Read the model definition and answer for the solid it produces. Units are mm, in the model's axes. Give positions to 0.01 mm unless a question says otherwise; leave off trailing zeros.
Autodesk Inventor part; units mm, degrees
ref_plane "YZ Plane" through (0, 0, 0) normal (1, 0, 0) x (0, 1, 0)
ref_plane "XZ Plane" through (0, 0, 0) normal (0, 1, 0) x (-1, 0, 0)
ref_plane "XY Plane" through (0, 0, 0) normal (0, 0, 1) x (1, 0, 0)
sketch "Sketch1" plane through (0, 0, 0) normal (0, 1, 0) x (-1, 0, 0)
  line L0 (69.85, 76.2) -> (-69.85, 76.2)
  line L1 (-69.85, 76.2) -> (-69.85, -76.2)
  line L2 (-69.85, -76.2) -> (69.85, -76.2)
  line L3 (69.85, -76.2) -> (69.85, 76.2)
  point P0 (0, 0)
  dimension "d0" = 152.4
  dimension "d1" = 139.7
  dimension "d2" = 69.85
  dimension "d3" = 76.2
extrude "Extrusion1" add sketch "Sketch1" along normal blind 12.7
sketch "Sketch4" plane through (0, 12.7, 0) normal (0, 1, 0) x (1, 0, 0)
  circle A0 centre (63.5, 69.85) radius 3.175
  circle A1 centre (63.5, -69.85) radius 3.175
  circle A2 centre (-60.96, -52.07) radius 3.175
  line L0 (69.85, 76.2) -> (-69.85, 76.2)
  line L1 (69.85, -76.2) -> (69.85, 76.2)
  line L2 (-69.85, -76.2) -> (69.85, -76.2)
  line L3 (-69.85, 76.2) -> (-69.85, -76.2)
  circle A3 centre (-60.96, 52.07) radius 3.175
  point P0 (0, 0)
  dimension "d20" = 6.35
  dimension "d21" = 6.35
  dimension "d22" = 6.35
  dimension "d23" = 6.35
  dimension "d24" = 6.35
  dimension "d25" = 6.35
  dimension "d26" = 6.35
  dimension "d27" = 24.13
  dimension "d28" = 8.89
  dimension "d32" = 6.35
  dimension "d33" = 24.13
  dimension "d34" = 8.89
extrude "Extrusion6" [suppressed]
fillet "Fillet1" [suppressed]
sketch "Sketch7" plane through (0, 12.7, 0) normal (0, 1, 0) x (1, 0, 0)
  arc A0 (-69.85, -37.0366) -> (-18.2851, -76.2) centre (46.0045, 61.976) ccw
  line L0 (69.85, 76.2) -> (-69.85, 76.2)
  line L1 (69.85, -76.2) -> (69.85, 76.2)
  line L2 (-69.85, 76.2) -> (-69.85, -76.2)
  line L3 (-69.85, -76.2) -> (69.85, -76.2)
  line L4 (-69.85, 76.2) -> (-69.85, -76.2)
  arc A1 (-18.2851, -76.2) -> (-69.85, -37.0366) centre (46.0045, 61.976) ccw
  point P0 (0, 0)
  point P1 (76.2, -60.325)
  point P2 (73.025, -60.325)
  point P3 (73.025, 63.5)
  point P4 (73.025, 60.325)
  point P5 (-73.025, 63.5)
  point P6 (76.2, 60.325)
  point P7 (73.025, -63.5)
  point P8 (-76.2, 60.325)
  point P9 (-80.9955, -22.2663)
  dimension "d46" = 304.8
  dimension "d47" = 14.224
  dimension "d48" = 23.8455
sketch "Sketch8" plane through (0, 12.7, 0) normal (0, 1, 0) x (1, 0, 0)
  circle A0 centre (-47.526, 0.6694) radius 1.4224
  circle A1 centre (-47.526, 0.6694) radius 1.4224
  circle A2 centre (-38.506, 0.6694) radius 1.4224
  line L0 (-33.996, -2.3847) -> (-52.036, -2.3847)
  line L1 (-33.996, 3.7235) -> (-33.996, -2.3847)
  line L2 (-33.996, 3.7235) -> (-52.036, 3.7235)
  line L3 (-52.036, -2.3847) -> (-52.036, 3.7235)
  circle A3 centre (-47.526, 33.9312) radius 1.4224
  circle A4 centre (-38.506, 33.9312) radius 1.4224
  line L4 (-33.996, 30.877) -> (-52.036, 30.877)
  line L5 (-33.996, 36.9853) -> (-33.996, 30.877)
  line L6 (-33.996, 36.9853) -> (-52.036, 36.9853)
  line L7 (-52.036, 30.877) -> (-52.036, 36.9853)
  circle A5 centre (2.54, -39.6875) radius 3.175 construction
  circle A6 centre (2.54, 12.7127) radius 3.175 construction
  circle A7 centre (2.54, 65.1129) radius 3.175 construction
  circle A8 centre (68.58, 65.1129) radius 3.175 construction
  circle A9 centre (68.58, 12.7127) radius 3.175 construction
  circle A10 centre (68.58, -39.6875) radius 3.175 construction
  circle A11 centre (-32.4275, -33.782) radius 1.4224
  circle A12 centre (-39.1585, -27.051) radius 1.4224
  circle A13 centre (-45.8895, -33.782) radius 1.4224
  circle A14 centre (-45.8895, 67.818) radius 1.4224
  circle A15 centre (-39.1585, 61.087) radius 1.4224
  circle A16 centre (-32.4275, 67.818) radius 1.4224
extrude "Extrusion9" cut sketch "Sketch8" against normal through all contours A0 | A2 | A3 | A4 | A11 | A12 | A13 | A14 | A15 | A16
extrude "Extrusion11" cut sketch "Sketch7" against normal through all contours A0 L3 L2
sketch "Sketch10" plane through (0, 12.7, 0) normal (0, 1, 0) x (1, 0, 0)
  circle A0 centre (62.611, 72.39) radius 1.4732
  arc A1 (-69.85, -37.0366) -> (-18.2851, -76.2) centre (46.0045, 61.976) ccw
  line L0 (-18.2851, -76.2) -> (69.85, -76.2)
  line L1 (69.85, -76.2) -> (69.85, 76.2)
  line L2 (69.85, 76.2) -> (-69.85, 76.2)
  line L3 (-69.85, 76.2) -> (-69.85, -37.0366)
  circle A2 centre (-47.526, 33.9312) radius 1.4224
  circle A3 centre (-47.526, 0.6694) radius 1.4224
  circle A4 centre (-38.506, 0.6694) radius 1.4224
  circle A5 centre (-38.506, 33.9312) radius 1.4224
  circle A6 centre (33.655, 72.39) radius 1.4732
  circle A7 centre (48.133, 72.39) radius 1.4732
  circle A8 centre (19.177, 72.39) radius 1.4732
  circle A9 centre (4.699, 72.39) radius 1.4732
  circle A10 centre (62.611, -68.58) radius 1.4732
  circle A11 centre (48.133, -68.58) radius 1.4732
  circle A12 centre (33.655, -68.58) radius 1.4732
  circle A13 centre (19.177, -68.58) radius 1.4732
  circle A14 centre (4.699, -68.58) radius 1.4732
  point P0 (0, 0)
extrude "Extrusion13" cut sketch "Sketch10" against normal through all contours A0 | A6 | A7 | A8 | A9 | A10 | A11 | A12 | A13 | A14
sketch "Sketch11" plane through (0, 12.7, 0) normal (0, 1, 0) x (1, 0, 0)
  circle A0 centre (19.177, 72.39) radius 1.4732
  circle A1 centre (48.133, 72.39) radius 1.4732
  circle A2 centre (62.611, -68.58) radius 1.4732
  circle A3 centre (33.655, -68.58) radius 1.4732
  circle A4 centre (4.699, -68.58) radius 1.4732
  circle A5 centre (1.27, -42.545) radius 1.4732
  circle A6 centre (1.27, -12.9117) radius 1.4732
  circle A7 centre (1.27, 16.7217) radius 1.4732
  circle A8 centre (1.27, 46.355) radius 1.4732
  circle A9 centre (66.04, 61.1717) radius 1.4732
  circle A10 centre (66.04, 31.5383) radius 1.4732
  circle A11 centre (66.04, 1.905) radius 1.4732
  circle A12 centre (66.04, -27.7283) radius 1.4732
  circle A13 centre (66.04, -57.3617) radius 1.4732
  circle A14 centre (66.04, -42.545) radius 1.4732
  circle A15 centre (66.04, -12.9117) radius 1.4732
  circle A16 centre (66.04, 16.7217) radius 1.4732
  circle A17 centre (66.04, 46.355) radius 1.4732
  circle A18 centre (1.27, 61.1717) radius 1.4732
  circle A19 centre (1.27, 31.5383) radius 1.4732
  circle A20 centre (1.27, 1.905) radius 1.4732
  circle A21 centre (1.27, -27.7283) radius 1.4732
  circle A22 centre (1.27, -57.3617) radius 1.4732
  circle A23 centre (19.177, -68.58) radius 1.4732
  circle A24 centre (48.133, -68.58) radius 1.4732
  circle A25 centre (62.611, 72.39) radius 1.4732
  circle A26 centre (33.655, 72.39) radius 1.4732
  circle A27 centre (4.699, 72.39) radius 1.4732
  line L0 (0.635, -72.39) -> (66.675, -72.39)
  line L1 (69.85, -69.215) -> (69.85, 73.025)
  line L2 (66.675, 76.2) -> (0.635, 76.2)
  line L3 (-2.54, 73.025) -> (-2.54, -69.215)
  arc A28 (59.055, 62.23) -> (55.88, 65.405) centre (55.88, 62.23) ccw
  line L4 (59.055, -58.42) -> (59.055, 62.23)
  arc A29 (55.88, -61.595) -> (59.055, -58.42) centre (55.88, -58.42) ccw
  line L5 (11.43, -61.595) -> (55.88, -61.595)
  arc A30 (8.255, -58.42) -> (11.43, -61.595) centre (11.43, -58.42) ccw
  line L6 (8.255, 62.23) -> (8.255, -58.42)
  arc A31 (11.43, 65.405) -> (8.255, 62.23) centre (11.43, 62.23) ccw
  line L7 (55.88, 65.405) -> (11.43, 65.405)
  arc A32 (69.85, 73.025) -> (66.675, 76.2) centre (66.675, 73.025) ccw
  arc A33 (0.635, 76.2) -> (-2.54, 73.025) centre (0.635, 73.025) ccw
  arc A34 (-2.54, -69.215) -> (0.635, -72.39) centre (0.635, -69.215) ccw
  arc A35 (66.675, -72.39) -> (69.85, -69.215) centre (66.675, -69.215) ccw
  point P0 (0, 0)
  point P1 (52.705, -61.595)
extrude "Extrusion14" cut sketch "Sketch11" against normal through all contours A5 | A6 | A7 | A8 | A9 | A10 | A11 | A12 | A13 | A14 | A15 | A16 | A17 | A18 | A19 | A20 | A21 | A22 | A25
sketch "Sketch14" plane through (0, 0, 0) normal (0, -1, 0) x (1, 0, 0)
  line L0 (69.85, -76.2) -> (-69.85, -76.2)
  line L1 (-18.2851, 76.2) -> (69.85, 76.2)
  circle A0 centre (4.699, -72.39) radius 1.4732
  circle A1 centre (-32.4275, -67.818) radius 1.4224
  point P0 (0, 0)
  point P1 (-13.8642, 44.45)
  point P2 (-13.8642, -44.45)
  dimension "d79" = 44.45
  dimension "d80" = 152.4
  dimension "d81" = 44.45
  dimension "d82" = 37.1265
  dimension "d83" = 18.5633
  dimension "d84" = 18.5633
hole "Hole2" at (-13.8642, 0, 44.45) at (-13.8642, 0, -44.45) direction (0, 1, 0) diameter 3.9624 end through all
sketch "Sketch15" plane through (0, 0, 0) normal (0, -1, 0) x (1, 0, 0)
  circle A0 centre (-13.8642, 44.45) radius 1.9812
  circle A1 centre (-13.8642, -44.45) radius 1.9812
  circle A2 centre (66.04, -31.5383) radius 1.4732
  circle A3 centre (1.27, -31.5383) radius 1.4732
  circle A4 centre (1.27, 42.545) radius 1.4732
  point P0 (0, 0)
  point P1 (33.655, -44.45)
  point P2 (33.655, 44.45)
  point P3 (33.655, 0)
  dimension "d92" = 44.45
  dimension "d93" = 44.45
  dimension "d94" = 44.45
  dimension "d95" = 44.45
  dimension "d96" = 64.77
  dimension "d97" = 32.385
  dimension "d98" = 32.385
  dimension "d222" = 32.385
  dimension "d223" = 44.45
hole "Hole3" at (33.655, 0, -44.45) at (33.655, 0, 44.45) at (33.655, 0, 0) direction (0, 1, 0) diameter 3.9624 depth 9.525
thread "Thread3"
thread "Thread4"
thread "Thread5"
thread "Thread6"
thread "Thread7"
thread "Thread8"
thread "Thread9"
thread "Thread10"
thread "Thread11"
thread "Thread12"
thread "Thread13"
thread "Thread14"
thread "Thread15"
thread "Thread16"
thread "Thread17"
thread "Thread18"
thread "Thread19"
thread "Thread20"
thread "Thread21"
thread "Thread22"
thread "Thread23"
thread "Thread24"
thread "Thread25"
thread "Thread26"
thread "Thread27"
thread "Thread28"
thread "Thread29"
thread "Thread30"
thread "Thread31"
thread "Thread32"
thread "Thread33"
thread "Thread34"
thread "Thread35"
thread "Thread36"
thread "Thread37"
thread "Thread38"
thread "Thread39"
thread "Thread40"
thread "Thread41"
sketch "Sketch16" plane through (0, 0, 0) normal (0, -1, 0) x (1, 0, 0)
  line L0 (-18.2851, 76.2) -> (69.85, 76.2)
  line L1 (69.85, -76.2) -> (-69.85, -76.2)
  line L2 (69.85, 76.2) -> (63.5, 76.2)
  line L3 (63.5, 76.2) -> (63.5, -76.2)
  line L4 (63.5, -76.2) -> (69.85, -76.2)
  line L5 (69.85, -76.2) -> (69.85, 76.2)
  point P0 (0, 0)
  dimension "d196" = 6.35
extrude "Extrusion15" [suppressed]
sketch "Sketch17" plane through (0, 12.7, 0) normal (0, 1, 0) x (1, 0, 0)
  line L0 (-48.26, -57.7736) -> (-69.85, -25.6538)
  line L1 (-69.85, 76.2) -> (-69.85, -37.0366)
  line L2 (-69.85, -25.6538) -> (-69.85, -37.0366)
  arc A0 (-69.85, -37.0366) -> (-18.2851, -76.2) centre (46.0045, 61.976) ccw
  arc A1 (-69.85, -37.0366) -> (-48.26, -57.7736) centre (46.0045, 61.976) ccw
  point P0 (0, 0)
  dimension "d200" = 6.35
  dimension "d203" = 21.59
extrude "Extrusion16" cut sketch "Sketch17" against normal through all
thread "Thread46"
thread "Thread47"
thread "Thread48"
sketch "Sketch19" plane through (0, 12.7, 0) normal (0, 1, 0) x (1, 0, 0)
  point P0 (0, 0)
  point P1 (-28.9602, -57.9611)
sketch "Sketch20" plane through (0, 0, 0) normal (0, -1, 0) x (1, 0, 0)
  circle A0 centre (-47.6269, -48.133) radius 2.3495
  circle A1 centre (-47.6269, 14.097) radius 2.3495
  point P0 (0, 0)
sketch "Sketch18" plane through (0, 12.7, 0) normal (0, 1, 0) x (1, 0, 0)
  circle A0 centre (-47.6269, -14.097) radius 2.794
  circle A1 centre (-47.6269, 48.133) radius 2.794
  point P0 (0, 0)
  point P1 (-53.9769, 60.833)
  point P2 (-53.9769, -26.797)
  dimension "d211" = 12.7
  dimension "d212" = 12.7
  dimension "d213" = 6.35
  dimension "d214" = 6.35
hole "Hole4" at (-53.9769, 12.7, -60.833) at (-53.9769, 12.7, 26.797) direction (0, -1, 0) diameter 3.9624 depth 12.7
sketch "Sketch21" plane through (0, 12.7, 0) normal (0, 1, 0) x (1, 0, 0)
  line L0 (69.85, 76.2) -> (-69.85, 76.2)
  line L1 (-69.85, 76.2) -> (-69.85, -25.6538)
  point P0 (0, 0)
  point P1 (-53.9242, -13.1826)
  point P2 (-40.9194, -13.1826)
  point P3 (-40.9194, 47.1932)
  point P4 (-53.9242, 47.1932)
  dimension "d224" = 29.0068
  dimension "d225" = 15.9258
  dimension "d226" = 28.9306
  dimension "d227" = 29.0068
  dimension "d228" = 15.9258
  dimension "d229" = 89.3826
  dimension "d230" = 89.3826
  dimension "d231" = 28.9306
hole "Hole5" at (-53.9242, 12.7, 13.1826) at (-40.9194, 12.7, 13.1826) at (-53.9242, 12.7, -47.1932) at (-40.9194, 12.7, -47.1932) direction (0, -1, 0) diameter 2.8448 end through all
equation "\"d21\" = d20"
equation "\"d22\" = d20"
equation "\"d24\" = d23"
equation "\"d25\" = d24"
equation "\"d26\" = d23"
equation "\"d32\" = d20"
equation "\"d33\" = d27"
equation "\"d34\" = d28"
properties part number "Base Plate Mk 2" material "Aluminum 6061"
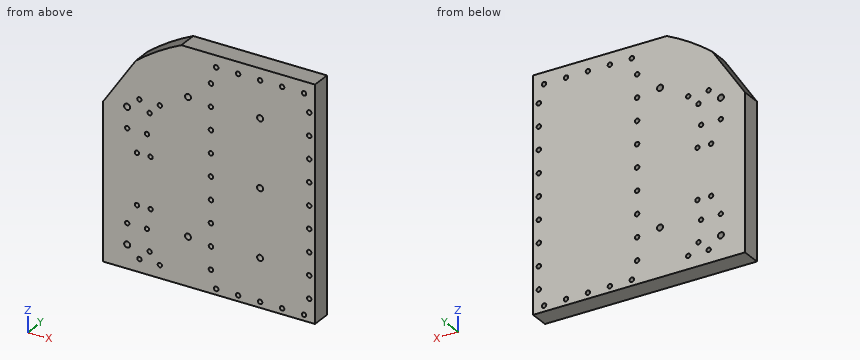
Item 1: Section A-A (y = 6) is taken. Give the number of separate pieces and of enclosed holes in the cut face, and give its area (3 significant figures).
Result set:
separate pieces: 1
enclosed holes: 49
area: 19,900 mm2
Item 2: Each of these flat-tipped pins is pushed along its axis until it touches: pin 1 Ø4.5 at (x, z) = (-53.92, 13.18) entering from +Y; pin 2 Ø5 at (y, z) = (6.5, 30.5) entering from -X; pin 3 Ø2.5 at (x, z) = (33.655, 0) entering from -Y (3 decimals). Where does it stop, or does it pass through?
Result set:
pin 1: stops at y = 12.7
pin 2: stops at x = -68.27
pin 3: stops at y = 9.525
Item 3: Find the intervals of material crossed by line 1 along Z through (x, y) = (19.5, 9); line 2 along X through (y, z) = (6.5, 43.5); line 3 along X through (y, z) = (5.75, -43), in increasing order.
Result set:
line 1: z = -76.2 to -73.83, -70.95 to 67.14, 70.02 to 76.2
line 2: x = -57.85 to -15.6, -12.13 to 0.15, 2.39 to 31.92, 35.39 to 64.92, 67.16 to 69.85
line 3: x = -69.85 to -15.21, -12.51 to 32.3, 35.01 to 69.85
